Could you check a few things on this model? Use its own coordinates, in mm. Give positions to 0.01 mm unless a question says otherwise; leave off trailing zeros. Order: outer loops, then holes, each group sorted by start corner. A loop starts at its lowest first (then second) coordinate and runs counter-clockwise, first axis right, second up.
(1) Imagine slicing it at C-C, the plane z = -5.5. Write out the boundary of the cut face in (x, y) (3 decimals).
(2) Imagine slicing it at D-D, the plane y = 14. Write out the boundary of the cut face in (x, z).
(3) Will these pins go through, and if not, where does the flat tip stop? pin 1 (1 mm diameter, centred on y = -15, z = -3, fed in from +X); pin 2 (10 mm diameter, centred on y = 9, z = -0.5, fed in from +X); pin 3 (5 mm diameter, centred on x = 7, z = -5, fed in from +Y).
(4) If I drill on probe 1 along Y at (x, z) = (0, -0.25) (3 decimals); probe 2 along Y at (x, z) = (0, 6); probe 3 along X at (y, z) = (1, 9.5), over which ranges is the centre line in solid material (lowest first)?
(5) Imagine slicing it at A-A, the plane y = 0. Write out the boundary of the cut face in (x, z) (3 decimals).
(6) If we mould it in two halves opening along X, with no side actions, what happens to faces 1 (the cylindrical face through (-3.441, -15.497, -6.261)), 2 (the cylindrical face through (-1.38, -6.2, 0.18)), 3 (the flat face through (-4, 16, 0))? For each: released by +X, released by -X, zero draft, split by the parting line, or undercut.
Autodesk Inventor part; units mm, degrees
ref_plane "YZ Plane" through (0, 0, 0) normal (1, 0, 0) x (0, 1, 0)
ref_plane "XZ Plane" through (0, 0, 0) normal (0, 1, 0) x (-1, 0, 0)
ref_plane "XY Plane" through (0, 0, 0) normal (0, 0, 1) x (1, 0, 0)
sketch "Sketch1" plane through (0, 0, 0) normal (0, 0, 1) x (1, 0, 0)
  circle A0 centre (0, 0) radius 19.05
  circle A1 centre (0, 0) radius 15.875
  circle A2 centre (0, 0) radius 6.35
  dimension "d0" = 38.1
  dimension "d1" = 31.75
  dimension "d2" = 12.7
extrude "Extrusion1" add sketch "Sketch1" against normal blind 12.7 contours A1
extrude "Extrusion2" add sketch "Sketch1" along normal blind 12.7 contours A0 | A1
properties part number "smaller gear"
Answer block:
1. outline: circle Ø31.75 at (0, 0); hole circle Ø12.7 at (0, 0)
2. outline: (-12.92, 0) - (-7.48, 0) - (-7.48, -12.7) - (7.48, -12.7) - (7.48, 0) - (12.92, 0) - (12.92, 12.7) - (-12.92, 12.7) - close
3. pin 1: stops at x = 6.46
3. pin 2: stops at x = 18.62
3. pin 3: stops at y = 15.22
4. probe 1: y = -15.875 to -6.35, 6.35 to 15.875
4. probe 2: y = -19.05 to -6.35, 6.35 to 19.05
4. probe 3: x = -19.02 to -6.27, 6.27 to 19.02
5. outline: (-19.05, 0) - (-15.875, 0) - (-15.875, -12.7) - (-6.35, -12.7) - (-6.35, 12.7) - (-19.05, 12.7) - close; (6.35, -12.7) - (15.875, -12.7) - (15.875, 0) - (19.05, 0) - (19.05, 12.7) - (6.35, 12.7) - close
6. face 1: split by the parting line
6. face 2: undercut
6. face 3: zero draft
